Verification items for the finished model (mm, model axes). Face numbers are marked on the shaded views. A direction names the side the tool comes from. Coordinates: 2 decimals unless noted, no trailing zeros. Order: outer loops, then holes, each group sorted by start corner. A loop starts at its lowest first (then second) coordinate and runs counter-clockwise, first axis right, second up.
Q1. Thickness scan on line 1 (X direction, y = 3.05, z = 5.25); line 2 (Z direction, x = -5.5, y = 4); line 3 (X direction, y = 2.7, z = 0). Record the ranges inside material, lowest first.
Q2. Depth check by flat-ended pin: P1, Ø1, axis at x = -1, z = -0.5, coming from the -Y side. Enter the tip coordinate at first touch or a pass-through.
Q3. Draft check along Z on the marked faces 5, 6 and 7. Enter one of: pulls with the +Z half, pulls with the -Z half, needs draft (parallel to the pull), parting line crosses it, or undercut.
Q4. Cross-section at A-A, the plane x = -0.5. Record the boundary of the cut face in (y, z).
Q5. Set-up check for the marked faces 1, 2, 3 and 4: record each of +Z, -Z, +X, -X, +Y, -Y from which the full face is reachable in a straight line by a thin tool's end or side.
Q6. Cross-section at B-B, the plane z = 0. Record the boundary of the cut face in (x, y).
from build123d import *

# Parameters (mm, degrees)
SKETCH1_R           = 3.25
BOSS_EXTRUDE2_DEPTH = 6
FILLET1_R           = 0.35


with BuildPart() as part:
    # Sketch1 → Boss-Extrude2 (new body)
    with BuildSketch(Plane(origin=(0, 0, 0), x_dir=(1, 0, 0), z_dir=(0, 1, 0))):
        with BuildLine():
            Line((1, 4.898979486), (0, 7))
            Line((0, 7), (-1, 4.898979486))
            ThreePointArc((-1, 4.898979486), (-1.039558454, 4.890738004), (-1.079049013, 4.882177099))
            Line((-1.079049013, 4.882177099), (-2.847156502, 6.394818203))
            Line((-2.847156502, 6.394818203), (-2.906139928, 4.068703813))
            ThreePointArc((-2.906139928, 4.068703813), (-2.938926261, 4.045084972), (-2.971520648, 4.021201939))
            Line((-2.971520648, 4.021201939), (-5.202013778, 4.683914245))
            Line((-5.202013778, 4.683914245), (-4.309781861, 2.534912288))
            ThreePointArc((-4.309781861, 2.534912288), (-4.330127019, 2.5), (-4.350189369, 2.464924432))
            Line((-4.350189369, 2.464924432), (-6.657395614, 2.163118961))
            Line((-6.657395614, 2.163118961), (-4.968223357, 0.5628114))
            ThreePointArc((-4.968223357, 0.5628114), (-4.972609477, 0.522642316), (-4.976670827, 0.482439098))
            Line((-4.976670827, 0.482439098), (-6.961653268, -0.731699243))
            Line((-6.961653268, -0.731699243), (-4.7676139, -1.506604693))
            ThreePointArc((-4.7676139, -1.506604693), (-4.755282581, -1.545084972), (-4.742640687, -1.583464339))
            Line((-4.742640687, -1.583464339), (-6.062177826, -3.5))
            Line((-6.062177826, -3.5), (-3.742640687, -3.315515147))
            ThreePointArc((-3.742640687, -3.315515147), (-3.715724127, -3.345653032), (-3.688564887, -3.375572407))
            Line((-3.688564887, -3.375572407), (-4.114496766, -5.663118961))
            Line((-4.114496766, -5.663118961), (-2.070530899, -4.551142911))
            ThreePointArc((-2.070530899, -4.551142911), (-2.033683215, -4.567727288), (-1.996702709, -4.584013339))
            Line((-1.996702709, -4.584013339), (-1.455381836, -6.847033205))
            Line((-1.455381836, -6.847033205), (-0.040407507, -4.999836721))
            ThreePointArc((-0.040407507, -4.999836721), (0, -5), (0.040407507, -4.999836721))
            Line((0.040407507, -4.999836721), (1.455381836, -6.847033205))
            Line((1.455381836, -6.847033205), (1.996702709, -4.584013339))
            ThreePointArc((1.996702709, -4.584013339), (2.033683215, -4.567727288), (2.070530899, -4.551142911))
            Line((2.070530899, -4.551142911), (4.114496766, -5.663118961))
            Line((4.114496766, -5.663118961), (3.688564887, -3.375572407))
            ThreePointArc((3.688564887, -3.375572407), (3.715724127, -3.345653032), (3.742640687, -3.315515147))
            Line((3.742640687, -3.315515147), (6.062177826, -3.5))
            Line((6.062177826, -3.5), (4.742640687, -1.583464339))
            ThreePointArc((4.742640687, -1.583464339), (4.755282581, -1.545084972), (4.7676139, -1.506604693))
            Line((4.7676139, -1.506604693), (6.961653268, -0.731699243))
            Line((6.961653268, -0.731699243), (4.976670827, 0.482439098))
            ThreePointArc((4.976670827, 0.482439098), (4.972609477, 0.522642316), (4.968223357, 0.5628114))
            Line((4.968223357, 0.5628114), (6.657395614, 2.163118961))
            Line((6.657395614, 2.163118961), (4.350189369, 2.464924432))
            ThreePointArc((4.350189369, 2.464924432), (4.330127019, 2.5), (4.309781861, 2.534912288))
            Line((4.309781861, 2.534912288), (5.202013778, 4.683914245))
            Line((5.202013778, 4.683914245), (2.971520648, 4.021201939))
            ThreePointArc((2.971520648, 4.021201939), (2.938926261, 4.045084972), (2.906139928, 4.068703813))
            Line((2.906139928, 4.068703813), (2.847156502, 6.394818203))
            Line((2.847156502, 6.394818203), (1.079049013, 4.882177099))
            ThreePointArc((1.079049013, 4.882177099), (1.039558454, 4.890738004), (1, 4.898979486))
        make_face()
        with Locations(Location((0, 0, 0), (0, 0, 270))):
            Circle(SKETCH1_R, mode=Mode.SUBTRACT)
    extrude(amount=BOSS_EXTRUDE2_DEPTH)

    # Fillet1
    fillet1_edges = [part.edges().sort_by_distance(p)[0] for p in [
        (2.847156502, 3, -6.394818203),
        (5.202013778, 3, -4.683914245),
        (6.657395614, 3, -2.163118961),
        (6.961653268, 3, 0.731699243),
        (6.062177826, 3, 3.5),
        (4.114496766, 3, 5.663118961),
        (1.455381836, 3, 6.847033205),
        (-1.455381836, 3, 6.847033205),
        (-4.114496766, 3, 5.663118961),
        (-6.062177826, 3, 3.5),
        (-6.961653268, 3, 0.731699243),
        (-6.657395614, 3, -2.163118961),
        (-5.202013778, 3, -4.683914245),
        (-2.847156502, 3, -6.394818203),
        (0, 3, -7),
    ]]
    fillet(fillet1_edges, radius=FILLET1_R)


solid = part.part
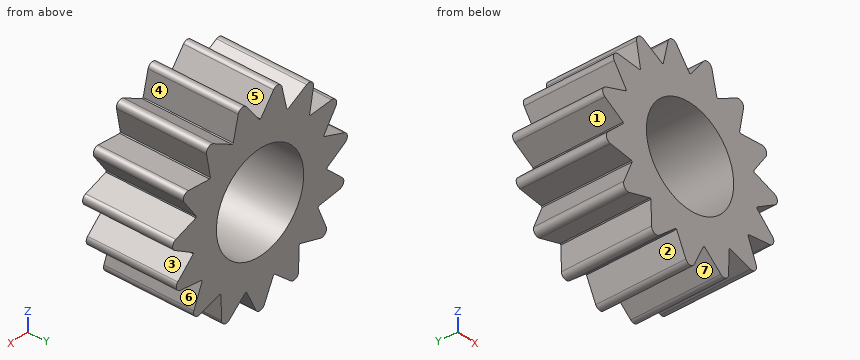
Check values:
1. line 1: x = -3.89 to -3.36, -1.84 to -0.23, 0.23 to 1.84, 3.36 to 3.89
1. line 2: z = -2.31 to -1.07, -0.16 to 1.25, 2.68 to 3.41
1. line 3: x = -5.77 to -3.25, 3.25 to 5.77
2. P1: passes through
3. face 5: pulls with the +Z half
3. face 6: undercut
3. face 7: pulls with the -Z half
4. outline: (0, -5.95) - (6, -5.95) - (6, -3.21) - (0, -3.21) - close; (0, 3.21) - (6, 3.21) - (6, 5.6) - (0, 5.6) - close
5. face 1: -X, +Y, -Y
5. face 2: -Z, +Y, -Y
5. face 3: +X, +Y, -Y
5. face 4: +Z, +Y, -Y
6. outline: (-5.77, 0) - (-3.25, 0) - (-3.25, 6) - (-5.77, 6) - close; (3.25, 0) - (5.77, 0) - (5.77, 6) - (3.25, 6) - close
